```python
from build123d import *

# Parameters (mm, degrees)
BOSS_EXTRUDE1_DEPTH = 10
CUT_EXTRUDE1_REACH  = 157.563
SKETCH2_R           = 2.5


with BuildPart() as part:
    # Sketch1 → Boss-Extrude1 (new body)
    with BuildSketch(Plane.XY):
        Polygon((0, 0), (40, 0), (40, 78.89880614), (30, 78.89880614), (30, 150), (-40, 150), (-40, 80), (-40, 40), align=None)
    extrude(amount=BOSS_EXTRUDE1_DEPTH)

    # Sketch2 → Cut-Extrude1 (cut, up to next)
    with BuildSketch(Plane.XY.offset(10), mode=Mode.PRIVATE) as cut_extrude1_sk1:
        with Locations((-30, 70)):
            Circle(SKETCH2_R)
    cut_extrude1_tool1 = extrude(cut_extrude1_sk1.sketch, amount=-CUT_EXTRUDE1_REACH, mode=Mode.PRIVATE) & part.part
    # Sketch2 → Cut-Extrude1 (cut, up to next)
    with BuildSketch(Plane.XY.offset(10), mode=Mode.PRIVATE) as cut_extrude1_sk2:
        with Locations((-10, 70)):
            Circle(SKETCH2_R)
    cut_extrude1_tool2 = extrude(cut_extrude1_sk2.sketch, amount=-CUT_EXTRUDE1_REACH, mode=Mode.PRIVATE) & part.part
    # Sketch2 → Cut-Extrude1 (cut, up to next)
    with BuildSketch(Plane.XY.offset(10), mode=Mode.PRIVATE) as cut_extrude1_sk3:
        with Locations((-30, 50)):
            Circle(SKETCH2_R)
    cut_extrude1_tool3 = extrude(cut_extrude1_sk3.sketch, amount=-CUT_EXTRUDE1_REACH, mode=Mode.PRIVATE) & part.part
    # Sketch2 → Cut-Extrude1 (cut, up to next)
    with BuildSketch(Plane.XY.offset(10), mode=Mode.PRIVATE) as cut_extrude1_sk4:
        with Locations((-10, 50)):
            Circle(SKETCH2_R)
    cut_extrude1_tool4 = extrude(cut_extrude1_sk4.sketch, amount=-CUT_EXTRUDE1_REACH, mode=Mode.PRIVATE) & part.part
    # Sketch2 → Cut-Extrude1 (cut, up to next)
    with BuildSketch(Plane.XY.offset(10), mode=Mode.PRIVATE) as cut_extrude1_sk5:
        with Locations((10, 50)):
            Circle(SKETCH2_R)
    cut_extrude1_tool5 = extrude(cut_extrude1_sk5.sketch, amount=-CUT_EXTRUDE1_REACH, mode=Mode.PRIVATE) & part.part
    # Sketch2 → Cut-Extrude1 (cut, up to next)
    with BuildSketch(Plane.XY.offset(10), mode=Mode.PRIVATE) as cut_extrude1_sk6:
        with Locations((30, 50)):
            Circle(SKETCH2_R)
    cut_extrude1_tool6 = extrude(cut_extrude1_sk6.sketch, amount=-CUT_EXTRUDE1_REACH, mode=Mode.PRIVATE) & part.part
    # Sketch2 → Cut-Extrude1 (cut, up to next)
    with BuildSketch(Plane.XY.offset(10), mode=Mode.PRIVATE) as cut_extrude1_sk7:
        with Locations((10, 10)):
            Circle(SKETCH2_R)
    cut_extrude1_tool7 = extrude(cut_extrude1_sk7.sketch, amount=-CUT_EXTRUDE1_REACH, mode=Mode.PRIVATE) & part.part
    # Sketch2 → Cut-Extrude1 (cut, up to next)
    with BuildSketch(Plane.XY.offset(10), mode=Mode.PRIVATE) as cut_extrude1_sk8:
        with Locations((30, 10)):
            Circle(SKETCH2_R)
    cut_extrude1_tool8 = extrude(cut_extrude1_sk8.sketch, amount=-CUT_EXTRUDE1_REACH, mode=Mode.PRIVATE) & part.part
    # Sketch2 → Cut-Extrude1 (cut, up to next)
    with BuildSketch(Plane.XY.offset(10), mode=Mode.PRIVATE) as cut_extrude1_sk9:
        with Locations((10, 90)):
            Circle(SKETCH2_R)
    cut_extrude1_tool9 = extrude(cut_extrude1_sk9.sketch, amount=-CUT_EXTRUDE1_REACH, mode=Mode.PRIVATE) & part.part
    # Sketch2 → Cut-Extrude1 (cut, up to next)
    with BuildSketch(Plane.XY.offset(10), mode=Mode.PRIVATE) as cut_extrude1_sk10:
        with Locations((10, 70)):
            Circle(SKETCH2_R)
    cut_extrude1_tool10 = extrude(cut_extrude1_sk10.sketch, amount=-CUT_EXTRUDE1_REACH, mode=Mode.PRIVATE) & part.part
    # Sketch2 → Cut-Extrude1 (cut, up to next)
    with BuildSketch(Plane.XY.offset(10), mode=Mode.PRIVATE) as cut_extrude1_sk11:
        with Locations((30, 70)):
            Circle(SKETCH2_R)
    cut_extrude1_tool11 = extrude(cut_extrude1_sk11.sketch, amount=-CUT_EXTRUDE1_REACH, mode=Mode.PRIVATE) & part.part
    add(cut_extrude1_tool1.solids().sort_by_distance((-30, 70, 10))[0], mode=Mode.SUBTRACT)
    add(cut_extrude1_tool2.solids().sort_by_distance((-10, 70, 10))[0], mode=Mode.SUBTRACT)
    add(cut_extrude1_tool3.solids().sort_by_distance((-30, 50, 10))[0], mode=Mode.SUBTRACT)
    add(cut_extrude1_tool4.solids().sort_by_distance((-10, 50, 10))[0], mode=Mode.SUBTRACT)
    add(cut_extrude1_tool5.solids().sort_by_distance((10, 50, 10))[0], mode=Mode.SUBTRACT)
    add(cut_extrude1_tool6.solids().sort_by_distance((30, 50, 10))[0], mode=Mode.SUBTRACT)
    add(cut_extrude1_tool7.solids().sort_by_distance((10, 10, 10))[0], mode=Mode.SUBTRACT)
    add(cut_extrude1_tool8.solids().sort_by_distance((30, 10, 10))[0], mode=Mode.SUBTRACT)
    add(cut_extrude1_tool9.solids().sort_by_distance((10, 90, 10))[0], mode=Mode.SUBTRACT)
    add(cut_extrude1_tool10.solids().sort_by_distance((10, 70, 10))[0], mode=Mode.SUBTRACT)
    add(cut_extrude1_tool11.solids().sort_by_distance((30, 70, 10))[0], mode=Mode.SUBTRACT)


solid = part.part
```
Could you check a few things on this model? Use its own coordinates, in mm. A direction names the side the tool comes from. Round coordinates to 2 decimals unless told otherwise and drop trailing zeros. Loops run counter-clockwise (first coordinate to the right, second up) from the corner with the lowest first, then second, coordinate; pieces in that order, holes last.
Q1. I want a section at C-C (z = 2). Give the number of separate pieces and of enclosed holes in the cut face, and give its area (3 significant figures).
Q2. I want a section at B-B (y = 50). Write out the boundary of the cut face in (x, z), and give its area (3 significant figures).
Q3. On a 3-axis mill with a long thin cutter (end or side, diameter ignored), from which of +Z, -Z, +X, -X, +Y, -Y can I reach the whole of each face in a straight line? I mean faces 4 (the cylindrical face through (-11.84, 51.69, 5.07)), 5 (the flat face through (30, 114, 5)). Say none if no direction works.
Q4. I want a section at D-D (x = -10). Write out the boundary of the cut face in (y, z).
Q5. I want a section at A-A (x = 10). Write out the boundary of the cut face in (y, z).
Q6. Please list where these lines run through material, in increasing order: L1, parallel to Y at x = 10, z = 7.75; L2, parallel to Y at x = -10, z = 4.75; L3, parallel to X at y = 48.5, z = 8.25.
Q7. Thinking about a two-plate mould opening in Y: for faces 1 (the flat face through (20, 0, 5)), 2 (the cylindrical face through (9.67, 92.48, 5.07)), 3 (the flat face through (-40, 96, 5)), which applies, pulls with the +Y half, pulls with the -Y half, needs draft (parallel to the pull), parting line crosses it, or undercut?
Q8. For P1, Ø4, axis at x = 10, y = 10, coming from the +Z side; P2, Ø6, axis at y = 27, z = 4, coming from the -X side; P3, Ø4, axis at y = 89, z = 9, coming from the +X side, each with a flat end and sliding along its axis, tell me the tip position at first contact or that it passes through.
Answer below:
1. separate pieces: 1
1. enclosed holes: 11
1. area: 10,300 mm2
2. outline: (-40, 0) - (-32.5, 0) - (-32.5, 10) - (-40, 10) - close; (-27.5, 0) - (-12.5, 0) - (-12.5, 10) - (-27.5, 10) - close; (-7.5, 0) - (7.5, 0) - (7.5, 10) - (-7.5, 10) - close; (12.5, 0) - (27.5, 0) - (27.5, 10) - (12.5, 10) - close; (32.5, 0) - (40, 0) - (40, 10) - (32.5, 10) - close
2. area: 600 mm2
3. face 4: +Z, -Z
3. face 5: +Z, -Z, +X, +Y
4. outline: (10, 0) - (47.5, 0) - (47.5, 10) - (10, 10) - close; (52.5, 0) - (67.5, 0) - (67.5, 10) - (52.5, 10) - close; (72.5, 0) - (150, 0) - (150, 10) - (72.5, 10) - close
5. outline: (0, 0) - (7.5, 0) - (7.5, 10) - (0, 10) - close; (12.5, 0) - (47.5, 0) - (47.5, 10) - (12.5, 10) - close; (52.5, 0) - (67.5, 0) - (67.5, 10) - (52.5, 10) - close; (72.5, 0) - (87.5, 0) - (87.5, 10) - (72.5, 10) - close; (92.5, 0) - (150, 0) - (150, 10) - (92.5, 10) - close
6. L1: y = 0 to 7.5, 12.5 to 47.5, 52.5 to 67.5, 72.5 to 87.5, 92.5 to 150
6. L2: y = 10 to 47.5, 52.5 to 67.5, 72.5 to 150
6. L3: x = -40 to -32, -28 to -12, -8 to 8, 12 to 28, 32 to 40
7. face 1: pulls with the -Y half
7. face 2: undercut
7. face 3: needs draft
8. P1: passes through
8. P2: stops at x = -30
8. P3: stops at x = 30
